Geometry: final body of the model. Coordinates: model frame, mm. A direction names the side the tool comes from. Give positions to 0.01 mm unless a question says otherwise; leave off trailing zeros. Order: outer loops, then holes, each group sorted by start corner. A loop starts at its lowest first (then second) coordinate and runs counter-clockwise, first axis right, second up. Notation, with made-up numbers: (-32.75, 69.5) - (-5.75, 69.5) arc R36 cw to (-5.75, 106.5) - close; hole circle Ø1 at (62, 79). An arc over 180 degrees is marked (long way). Use one line per item in the form item = value.
from build123d import *

# Parameters (mm, degrees)
F1_DEPTH = 2.4
F3_DEPTH = 17.61
F5_DEPTH = 2.8
F7_DEPTH = 16.06
F8_R     = 0.5


with BuildPart() as f1:
    # F0 (on Top) → F1 (new body, symmetric)
    with BuildSketch(Plane.XY):
        with BuildLine():
            ThreePointArc((10.47, 9.23), (9.8842135624, 10.6442135624), (8.47, 11.23))
            Line((8.47, 11.23), (-8.47, 11.23))
            ThreePointArc((-8.47, 11.23), (-9.8842135624, 10.6442135624), (-10.47, 9.23))
            Line((-10.47, 9.23), (-10.47, -11.23))
            Line((-10.47, -11.23), (10.47, -11.23))
            Line((10.47, -11.23), (10.47, 9.23))
        make_face()
    extrude(amount=F1_DEPTH, both=True)

    # F2 (on face) → F3 (join)
    with BuildSketch(Plane.XY.offset(2.4)):
        with BuildLine():
            ThreePointArc((-3.75, -3.025), (0, -6.775), (3.75, -3.025))
            Line((3.75, -3.025), (3.75, 3.025))
            Line((3.75, 3.025), (2.1, 7.325))
            Line((2.1, 7.325), (-2.1, 7.325))
            Line((-2.1, 7.325), (-3.75, 3.025))
            Line((-3.75, 3.025), (-3.75, -3.025))
        make_face()
    extrude(amount=F3_DEPTH)

    # F4 (on face) → F5 (cut)
    with BuildSketch(Plane(origin=(0, 0, -2.4), x_dir=(1, 0, 0), z_dir=(0, 0, -1))):
        Polygon((-5.72, 8.08), (-5.72, -7.98), (5.72, -7.98), (5.72, 8.08), (8.75, 8.08), (8.75, 11.23), (-8.75, 11.23), (-8.75, 8.08), align=None)
    extrude(amount=-F5_DEPTH, mode=Mode.SUBTRACT)

    # F6 (on face) → F7 (cut, through all)
    with BuildSketch(Plane.XZ.offset(8.08)):
        Polygon((-8.75, 0.4), (-5.72, -2.4), (-5.72, 0.4), align=None)
        Polygon((5.72, -2.4), (8.75, 0.4), (5.72, 0.4), align=None)
    extrude(amount=-F7_DEPTH, mode=Mode.SUBTRACT)

    # F8
    f8_edges = [f1.edges().sort_by_distance(p)[0] for p in [
        (10.47, -1, 2.4),
        (3.75, 3.025, 11.205),
        (-3.75, 3.025, 11.205),
        (-2.1, 7.325, 11.205),
        (2.1, 7.325, 11.205),
        (0, -6.775, 2.4),
        (9.884214, 10.644214, 2.4),
        (-10.47, -1, 2.4),
        (-9.884214, 10.644214, 2.4),
        (0, 11.23, 2.4),
        (3.75, 0, 2.4),
        (2.925, 5.175, 2.4),
        (0, 7.325, 2.4),
        (-2.925, 5.175, 2.4),
        (-3.75, 0, 2.4),
    ]]
    fillet(f8_edges, radius=F8_R)


solid = f1.part
(1) Contact query for flat-ended pins moving along their axis: pin 1 Ø0.8 at (x, z) = (7.5, -0.5) entering from -Y; pin 2 Ø2 at (x, z) = (-3, 11) entering from -Y; pin 3 Ø3 at (x, z) = (0.5, 12.5) entering from +Y (3 decimals). Output: stop coordinate, or through.
Computed values:
pin_1 = -8.08
pin_2 = -6.2
pin_3 = 7.325
(2) Reachability of faces 4 (the face through (-8, -8.08, -1)), 5 (the face through (-3.75, 0, 11)), 6 (the face through (0, 7.98, -1)), 7 (the face through (-0.082, -6.774, 11.335)), 8 (the face through (-2.96, 5.085, 11.335)) from +Z, -Z, +X, -X, +Y, -Y: full face, straight path, thin tool, end or side. Return the list, or none.
Computed values:
face_4 = -Z, -Y
face_5 = +Z, -X, +Y, -Y
face_6 = -Y
face_7 = +Z, -Y
face_8 = +Z, -X, +Y
(3) Ray query, line 1 along Z through (x, y) = (2.5, -1.5); line 2 along X through (y, z) = (-1.5, 13.75); line 3 along Z through (x, y) = (-2, -8.5). Return the intervals inside material, ascending.
Computed values:
line_1 = 0.4 to 20.01
line_2 = -3.75 to 3.75
line_3 = 0.4 to 2.4
(4) Cut plane C-C on x = 0. Output: boundary loops of the cut face in (y, z) (3 decimals).
Computed values:
outline = (-11.23, 0.4) - (7.98, 0.4) - (7.98, -2.4) - (11.23, -2.4) - (11.23, 1.9) arc R0.5 ccw to (10.73, 2.4) - (7.825, 2.4) arc R0.5 cw to (7.325, 2.9) - (7.325, 20.01) - (-6.775, 20.01) - (-6.775, 2.9) arc R0.5 cw to (-7.275, 2.4) - (-11.23, 2.4) - close
(5) Cut plane B-B on z = 15.5. Output: boundary loops of the cut face in (x, y) (3 decimals).
Computed values:
outline = (-3.75, -3.025) arc R3.75 ccw to (3.75, -3.025) - (3.75, 2.932) arc R0.5 ccw to (3.717, 3.111) - (2.223, 7.004) arc R0.5 ccw to (1.756, 7.325) - (-1.756, 7.325) arc R0.5 ccw to (-2.223, 7.004) - (-3.717, 3.111) arc R0.5 ccw to (-3.75, 2.932) - close
(6) Cut plane D-D on y = 8.75. Output: boundary loops of the cut face in (x, z).
Computed values:
outline = (-10.47, -2.4) - (10.47, -2.4) - (10.47, 1.9) arc R0.5 ccw to (9.97, 2.4) - (-9.97, 2.4) arc R0.5 ccw to (-10.47, 1.9) - close
(7) Cut plane A-A on y = -8.5. Output: boundary loops of the cut face in (x, z), plus the area to 3 significant figures.
Computed values:
outline = (-10.47, -2.4) - (-8.75, -2.4) - (-8.75, 0.4) - (8.75, 0.4) - (8.75, -2.4) - (10.47, -2.4) - (10.47, 1.9) arc R0.5 ccw to (9.97, 2.4) - (-9.97, 2.4) arc R0.5 ccw to (-10.47, 1.9) - close
area = 51.4 mm²
(8) Pull-direction query (X, two-part tool) for faces 1 (the face through (3.75, 0, 11)), 2 (the face through (-3.121, 5.084, 2.543)), 3 (the face through (-8.75, -10, -1)); classes: released by +X, released by -X, zero draft, split by the parting line, or undercut.
Computed values:
face_1 = released by +X
face_2 = released by -X
face_3 = undercut
